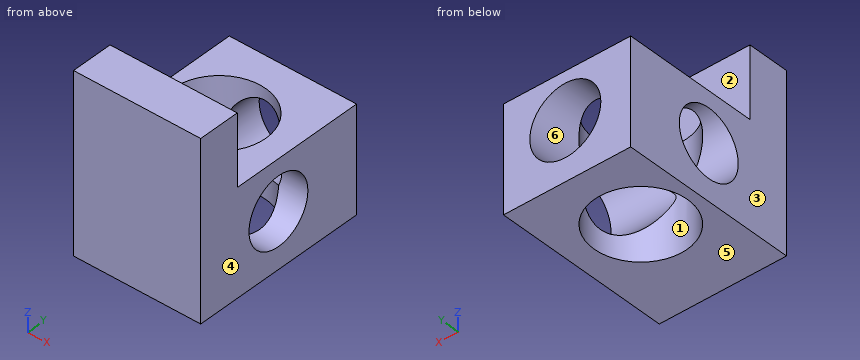
from build123d import *

# Parameters (mm, degrees)
F0_W      = 45.4768538475
F0_H      = 37.7318039536
F1_DEPTH  = 63.754
F2_R      = 16.6615499076
F3_DEPTH  = 75.184
F4_W      = 45.4768538475
F4_H      = 14.9607213655
F5_DEPTH  = 25.4
F8_R      = 12.0524100186
F10_DEPTH = 59.436
F11_R     = 12.7
F12_DEPTH = 25.4


# Not quite as in the source:
# - the program builds the solid bodies; features that only make, move or delete a surface that nothing else refers to are left out


with BuildPart() as f1:
    # F0 (on Front) → F1 (new body)
    with BuildSketch(Plane.XZ):
        with Locations((22.7384269238, 18.8659019768)):
            Rectangle(F0_W, F0_H)
    extrude(amount=F1_DEPTH)

    # F2 (on face) → F3 (cut)
    with BuildSketch(Plane.XY.offset(37.7318039536)):
        with Locations((20.3596297652, -27.4416878819)):
            Circle(F2_R)
    extrude(amount=-F3_DEPTH, mode=Mode.SUBTRACT)

    # F4 (on face) → F5 (join)
    with BuildSketch(Plane.XY.offset(37.7318039536)):
        with Locations((22.7384269238, -56.2736393173)):
            Rectangle(F4_W, F4_H)
    extrude(amount=F5_DEPTH)

    # F8 (on face) → F10 (cut)
    with BuildSketch(Plane.YZ.offset(45.4768538475)):
        with Locations((-31.9488979876, 19.8562797159)):
            Circle(F8_R)
    extrude(amount=-F10_DEPTH, mode=Mode.SUBTRACT)

    # F11 (on face) → F12 (cut)
    with BuildSketch(Plane(origin=(0, 0, 0), x_dir=(-1, 0, 0), z_dir=(0, 1, 0))):
        with Locations((-23.3701635152, 20.8852831274)):
            Circle(F11_R)
    extrude(amount=-F12_DEPTH, mode=Mode.SUBTRACT)


solid = f1.part
Work out the finished part from the listing and answer in its coordinate system (mm). Face numbers are marked on the shaded views. A direction names the side the tool comes from. Give positions to 0.01 mm unless a question says otherwise; leave off trailing zeros. Write each loop counter-clockwise with the first axis right and the second up, starting at its lowest first coordinate (ties: lowest second). Pieces come first, ordered by that corner, then holes. Notation, with made-up numbers: (-31.75, -29.75) - (-5.75, -29.75) arc R24 ccw to (-5.75, -6.75) - close; hole circle Ø1 at (72, -10.5). An arc over 180 degrees is marked (long way). One line per item, written item: value. Start each with the question number.
1. Consider probe 1 along Y at (x, z) = (27.5, 49.5); probe 2 along Z at (x, y) = (3, -29); probe 3 along X at (y, z) = (-20, 35.5). Determine where each line is inside the solid, lowest interval first.
2. Find section D-D (y = -12). Write down the section's boundary in (x, z).
3. For the marked faces 1 and 2, determine the directions among +Z, -Z, +X, -X, +Y, -Y from which every point of the face is accessible in a straight line to the end or side of a thin tool.
4. Given pin 1 (22.5 mm diameter, centred on x = 26, y = -33, fed in from +Z); pin 2 (8 mm diameter, centred on x = 23.5, z = 22.5, fed in from +Y), each flat-ended and moving along its own axis, determine where each tip first touches the part or whether it passes through.
5. Find section C-C (z = 12). Write down the section's boundary in (x, y).
6. Find section B-B (x = 32.5). Write down the section's boundary in (y, z), then the cut area to 3 significant figures.
7. For a pull along X with two mould halves and no side action, classify the marked faces 3, 4, 5 and 6 as +X half, -X half, draft (parallel to the pull), parting line (faces both ways), or undercut.
8. Find section A-A (y = -22). Write down the section's boundary in (x, z).
Geometry results:
1. probe 1: -63.75 to -48.79
1. probe 2: 0 to 8.17, 31.54 to 37.73
1. probe 3: 0 to 5.45, 35.27 to 45.48
2. outline: (0, 0) - (14.1, 0) - (14.1, 12.2) arc R12.7 cw to (14.1, 29.57) - (14.1, 37.73) - (0, 37.73) - close; (26.62, 0) - (45.48, 0) - (45.48, 37.73) - (26.62, 37.73) - (26.62, 33.16) arc R12.7 cw to (26.62, 8.61) - close
3. face 1: +Z, -Z
3. face 2: +Z, +X, -X, +Y
4. pin 1: z = 37.73
4. pin 2: y = -42.87
5. outline: (0, -63.75) - (45.48, -63.75) - (45.48, -41.09) - (29.92, -41.09) arc R16.66 cw to (10.8, -41.09) - (0, -41.09) - close; (0, -22.81) - (4.36, -22.81) arc R16.66 cw to (14.3, -11.92) - (14.3, 0) - (0, 0) - close; (32.44, -15.97) arc R16.66 cw to (36.36, -22.81) - (45.48, -22.81) - (45.48, 0) - (32.44, 0) - close
6. outline: (-63.75, 0) - (-38.85, 0) - (-38.85, 9.98) arc R12.05 cw to (-38.85, 29.74) - (-38.85, 37.73) - (-48.79, 37.73) - (-48.79, 63.13) - (-63.75, 63.13) - close; (-16.03, 0) - (0, 0) - (0, 12.06) - (-16.03, 12.06) - close; (-16.03, 29.71) - (0, 29.71) - (0, 37.73) - (-16.03, 37.73) - close
6. area: 1,570 mm2
7. face 3: -X half
7. face 4: +X half
7. face 5: draft
7. face 6: undercut
8. outline: (0, 0) - (4.61, 0) - (4.61, 13.05) - (0, 13.05) - close; (0, 26.66) - (4.61, 26.66) - (4.61, 37.73) - (0, 37.73) - close; (36.11, 0) - (45.48, 0) - (45.48, 13.05) - (36.11, 13.05) - close; (36.11, 26.66) - (45.48, 26.66) - (45.48, 37.73) - (36.11, 37.73) - close
